The listing builds one solid part. Answer for the finished solid, in the listing's coordinates (mm). Face numbers are marked on the shaded views. A direction names the side the tool comes from. Coordinates: 2 decimals unless noted, no trailing zeros. Order: outer loops, then holes, each group sorted by start corner. A loop starts at its lowest first (then second) coordinate and runs counter-clockwise, first axis right, second up. Notation, with made-up numbers: (61.25, 47) - (104.25, 47) arc R14 cw to (104.25, 60) - close; hole circle Ø1 at (-26, 9). An arc over 180 degrees is marked (long way). Use one line per item in the form item = value. Start each with the question number.
Item 1: Consider line 1 along Y through (x, z) = (9, 1.25); line 2 along X through (y, z) = (0, 3.25); line 3 along Z through (x, y) = (11.75, -2.5). Determine where each line is inside the solid, lowest interval first. Write a range as [from, to].
Item 2: Section A-A, the plane y = 0 is taken. Write down the section's boundary in (x, z).
Item 3: Section B-B, the plane z = 0 is taken. Write down the section's boundary in (x, y).
Item 4: A tool of negligible diameter and unlimited length cuts with its end or side. For the marked faces 1, 2 and 3, from which of +Z, -Z, +X, -X, +Y, -Y can it reach the whole face along a straight path? Write none if from no direction.
Item 5: Section D-D, the plane x = 11 is taken. Write down the section's boundary in (y, z), and give its area (3 significant figures).
Item 6: Each of these flat-tipped pins is pushed along its axis until it touches: pin 1 Ø1.5 at (y, z) = (-2, -3.5) entering from +X; pin 2 Ø3 at (x, y) = (8, 2.5) entering from -Z; pin 3 Ø4.5 at (x, y) = (10.5, 2) entering from +Z; pin 4 Ø5 at (y, z) = (-1, 2.5) entering from -X. Where does it stop, or does it pass through?
Item 7: Section C-C, the plane x = 7.75 is taken. Write down the section's boundary in (y, z).
from build123d import *

# Parameters (mm, degrees)
CUT_EXTRUDE1_DEPTH = 4


with BuildPart() as part:
    # Sketch1 → Revolve1 (revolve)
    with BuildSketch(Plane.XY):
        Polygon((0, 0), (0, 5), (8, 5), (12, 4), (12, 0), align=None)
    revolve(axis=Axis((12, 0, 0), (-1, 0, 0)))

    # Sketch2 → Cut-Extrude1 (cut)
    with BuildSketch(Plane(origin=(12, 0, 0), x_dir=(0, 0, -1), z_dir=(1, 0, 0))):
        with BuildLine():
            Line((-2, -3.464101615), (-2, 3.464101615))
            ThreePointArc((-2, 3.464101615), (-4, 0), (-2, -3.464101615))
        make_face()
        with BuildLine():
            Line((-2, 3.464101615), (-2, 4.582575695))
            ThreePointArc((-2, 4.582575695), (-5, 0), (-2, -4.582575695))
            Line((-2, -4.582575695), (-2, -3.464101615))
            ThreePointArc((-2, -3.464101615), (-4, 0), (-2, 3.464101615))
        make_face()
        with BuildLine():
            ThreePointArc((4, 0), (3.464101615, 2), (2, 3.464101615))
            Line((2, 3.464101615), (2, -3.464101615))
            ThreePointArc((2, -3.464101615), (3.464101615, -2), (4, 0))
        make_face()
        with BuildLine():
            ThreePointArc((5, 0), (4.183300133, 2.738612788), (2, 4.582575695))
            Line((2, 4.582575695), (2, 3.464101615))
            ThreePointArc((2, 3.464101615), (3.464101615, 2), (4, 0))
            ThreePointArc((4, 0), (3.464101615, -2), (2, -3.464101615))
            Line((2, -3.464101615), (2, -4.582575695))
            ThreePointArc((2, -4.582575695), (4.183300133, -2.738612788), (5, 0))
        make_face()
    extrude(amount=-CUT_EXTRUDE1_DEPTH, mode=Mode.SUBTRACT)


solid = part.part
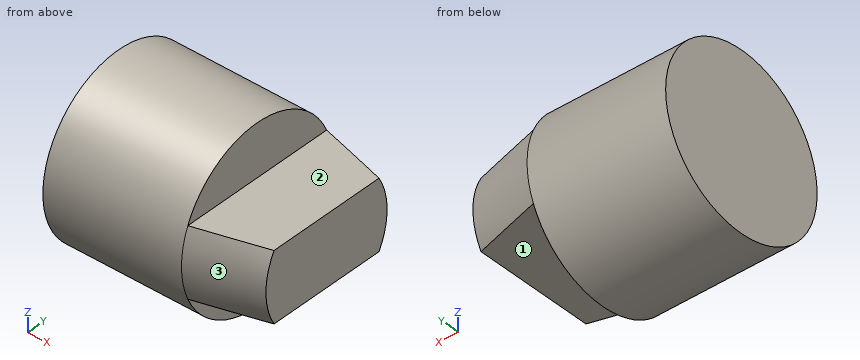
Response:
q1.line_1 = [-4.58, 4.58]
q1.line_2 = [0, 8]
q1.line_3 = [-2, 2]
q2.outline = (0, -5) - (8, -5) - (8, -2) - (12, -2) - (12, 2) - (8, 2) - (8, 5) - (0, 5) - close
q3.outline = (0, -5) - (8, -5) - (12, -4) - (12, 4) - (8, 5) - (0, 5) - close
q4.face_1 = -Z, +X, +Y, -Y
q4.face_2 = +Z, +X, +Y, -Y
q4.face_3 = +X, -Y
q5.outline = (-3.75, -2) - (3.75, -2) arc R4.25 ccw to (3.75, 2) - (-3.75, 2) arc R4.25 ccw to start
q5.area = 32.7 mm2
q6.pin_1 = 8
q6.pin_2 = -4.9
q6.pin_3 = 2
q6.pin_4 = 0
q7.outline = circle Ø10 at (0, 0)
